```python
from build123d import *
from build123d.topology import SkipClean

# Parameters (mm, degrees)
SKETCH1_R                = 10
BOSS_EXTRUDE1_DEPTH      = 20
SKETCH2_R                = 35
SKETCH2_R_2              = 25
BOSS_EXTRUDE2_DEPTH      = 20
BOSS_EXTRUDE3_START      = 30
SKETCH3_R                = 35
SKETCH3_R_2              = 25
BOSS_EXTRUDE3_DEPTH      = 30
SKETCH4_R                = 25
CUT_EXTRUDE1_DEPTH       = 131.862523283
BOSS_EXTRUDE6_REACH      = 176.428
BOSS_EXTRUDE6_END_RADIUS = 50
SKETCH6_W                = 75
SKETCH6_H                = 30
SKETCH7_W                = 65
SKETCH7_H                = 18
CUT_EXTRUDE2_DEPTH       = 40


with BuildPart() as part:
    # Sketch1 → Boss-Extrude1 (new, symmetric)
    with BuildSketch(Plane.XY):
        with BuildLine():
            Line((-85, 20), (-18.480117336, 46.459501324))
            ThreePointArc((-18.480117336, 46.459501324), (0, 50), (18.480117336, 46.459501324))
            Line((18.480117336, 46.459501324), (85, 20))
            ThreePointArc((85, 20), (105, 0), (85, -20))
            Line((85, -20), (18.480117336, -46.459501324))
            ThreePointArc((18.480117336, -46.459501324), (0, -50), (-18.480117336, -46.459501324))
            Line((-18.480117336, -46.459501324), (-85, -20))
            ThreePointArc((-85, -20), (-105, 0), (-85, 20))
        make_face()
        with Locations((-85, 0)):
            Circle(SKETCH1_R, mode=Mode.SUBTRACT)
        with Locations((85, 0)):
            Circle(SKETCH1_R, mode=Mode.SUBTRACT)
    extrude(amount=BOSS_EXTRUDE1_DEPTH, both=True)

    # Sketch2 → Boss-Extrude2 (add)
    with BuildSketch(Plane.XY.offset(20)):
        Circle(SKETCH2_R)
        Circle(SKETCH2_R_2, mode=Mode.SUBTRACT)
    extrude(amount=BOSS_EXTRUDE2_DEPTH)

    # Sketch3 → Boss-Extrude3 (add)
    with BuildSketch(Plane(origin=(0, 0, -20), x_dir=(-1, 0, 0), z_dir=(0, 0, -1)).offset(BOSS_EXTRUDE3_START)):
        with Locations(Location((0, 0, 0), (0, 0, 180))):
            Circle(SKETCH3_R)
        with Locations(Location((0, 0, 0), (0, 0, 180))):
            Circle(SKETCH3_R_2, mode=Mode.SUBTRACT)
    extrude(amount=-BOSS_EXTRUDE3_DEPTH)

    # Sketch4 → Cut-Extrude1 (cut, through all)
    with BuildSketch(Plane(origin=(0, 0, -20), x_dir=(-1, 0, 0), z_dir=(0, 0, -1))):
        Circle(SKETCH4_R)
    extrude(amount=-CUT_EXTRUDE1_DEPTH, mode=Mode.SUBTRACT)

    # Boss-Extrude6: up to this cylinder (the profile starts outside it)
    with SkipClean():  # the faces are left unmerged after this step: merging them gives an invalid solid
        boss_extrude6_end = Plane(origin=(0, 0, 0), z_dir=(0, 0, -1)) * Cylinder(BOSS_EXTRUDE6_END_RADIUS, 453.856, mode=Mode.PRIVATE)
        # Sketch6 → Boss-Extrude6 (add, up to the surface)
        with BuildSketch(Plane(origin=(0, 80, 0), x_dir=(1, 0, 0), z_dir=(0, 1, 0)), mode=Mode.PRIVATE) as boss_extrude6_sk1:
            Rectangle(SKETCH6_W, SKETCH6_H)
        boss_extrude6_tool1 = extrude(boss_extrude6_sk1.sketch, amount=-BOSS_EXTRUDE6_REACH, mode=Mode.PRIVATE) - boss_extrude6_end
        add(boss_extrude6_tool1.solids().sort_by_distance((0, 80, 0))[0])
    add(part.part.scale(1), mode=Mode.REPLACE)  # the faces are merged on a copy

    # Sketch7 → Cut-Extrude2 (cut)
    with BuildSketch(Plane(origin=(0, 80, 0), x_dir=(1, 0, 0), z_dir=(0, 1, 0))):
        Rectangle(SKETCH7_W, SKETCH7_H)
    extrude(amount=-CUT_EXTRUDE2_DEPTH, mode=Mode.SUBTRACT)


solid = part.part
```
Model file for the job. Use its own axes, mm. A direction names the side the tool comes from. Round coordinates to 2 decimals unless told otherwise and drop trailing zeros. Loops run counter-clockwise (first coordinate to the right, second up) from the corner with the lowest first, then second, coordinate; pieces in that order, holes last. Notation, with made-up numbers: M 29.5,-19 L 45.5,-19 A29 cw 45.5,18 Z; hole C 89.5,-21 d11. An arc over 180 degrees is marked long. Put each result on its own line as item: value. Start each with the question number.
Item 1: Drill centre lines: line 1 along X through (y, z) = (-1, -33); line 2 along Z through (x, y) = (-17, 68); line 3 along X through (y, z) = (5, -12). Where is each one in solid material? Low to high.
Item 2: Cut at C-C (y = 53). List the corners of the cut face in (x, z), then the cut area to 3 significant figures.
Item 3: Mould opens along Z. For faces 6 (the face through (-24, 8, 40)), 7 (the face through (75, 0, 0)), 8 (the face through (0, 60, -9)) say: released by +Z, released by -Z, zero draft, split by the parting line, or undercut.
Item 4: Cut at A-A (z = -5.5). List the corners of the cut face in (x, y), then the cut area to 3 significant figures.
Item 5: 3-axis set-ups, long thin cutter, end or side, ignore diameter. For faces 1 (the face through (-37.5, 60, 0)), 2 (the face through (-32.5, 60, 0)), 3 (the face through (0, 50, 18)), 4 (the face through (0, -50, 0)), 5 (the face through (37.5, 60, 0)): which of +Z, -Z, +X, -X, +Y, -Y reach the whole face in a straight line?
Item 6: Drop flat-ended pins along their axis: P1, Ø3, axis at x = -75.5, y = 7, coming from the +Z side; P2, Ø20, axis at y = 59, z = -2.5, coming from the -X side; P3, Ø4, axis at x = 4.5, y = 67, coming from the -Z side. Give the stop position or say it passes through.
Item 7: Cut at D-D (y = 15.5). List the corners of the cut face in (x, z), then the cut area to 3 significant figures.
Item 8: Cut at B-B (x = -3). List the corners of the cut face in (y, z), then the cut area to 3 significant figures.
Answer block:
1. line 1: -34.99 to -24.98, 24.98 to 34.99
1. line 2: -15 to -9, 9 to 15
1. line 3: -104.36 to -93.66, -76.34 to -24.49, 24.49 to 76.34, 93.66 to 104.36
2. outline: M -37.5,-15 L 37.5,-15 L 37.5,15 L -37.5,15 Z; hole M -32.5,-9 L 32.5,-9 L 32.5,9 L -32.5,9 Z
2. area: 1,080 mm2
3. face 6: released by +Z
3. face 7: zero draft
3. face 8: undercut
4. outline: M -85,-20 L -18.48,-46.46 A50 ccw 18.48,-46.46 L 85,-20 A20 ccw 85,20 L 37.5,38.89 L 37.5,80 L 32.5,80 L 32.5,40 L -32.5,40 L -32.5,80 L -37.5,80 L -37.5,38.89 L -85,20 A20 ccw Z; hole C -85,0 d20; hole C 0,0 d50; hole C 85,0 d20
4. area: 11,100 mm2
5. face 1: +Z, -Z, -X, +Y
5. face 2: +Y
5. face 3: +Z, +Y
5. face 4: +Z, -Z, -Y
5. face 5: +Z, -Z, +X, +Y
6. P1: z = 20
6. P2: x = -37.5
6. P3: z = -15
7. outline: M -97.64,-20 L -31.38,-20 L -31.38,-50 L -19.62,-50 L -19.62,40 L -31.38,40 L -31.38,20 L -97.64,20 Z; M 19.62,-50 L 31.38,-50 L 31.38,-20 L 97.64,-20 L 97.64,20 L 31.38,20 L 31.38,40 L 19.62,40 Z
7. area: 7,420 mm2
8. outline: M -49.91,-20 L -34.87,-20 L -34.87,-50 L -24.82,-50 L -24.82,40 L -34.87,40 L -34.87,20 L -49.91,20 Z; M 24.82,-50 L 34.87,-50 L 34.87,-20 L 49.91,-20 L 49.91,-15 L 80,-15 L 80,-9 L 40,-9 L 40,9 L 80,9 L 80,15 L 49.91,15 L 49.91,20 L 34.87,20 L 34.87,40 L 24.82,40 Z
8. area: 3,200 mm2
